Autodesk Inventor part; units mm, degrees
ref_plane "YZ Plane" through (0, 0, 0) normal (1, 0, 0) x (0, 1, 0)
ref_plane "XZ Plane" through (0, 0, 0) normal (0, 1, 0) x (-1, 0, 0)
ref_plane "XY Plane" through (0, 0, 0) normal (0, 0, 1) x (1, 0, 0)
sketch "Sketch1" plane through (0, 0, 0) normal (0, 0, 1) x (1, 0, 0)
  line L0 (-20, -7.5) -> (20, -7.5)
  line L1 (20, -7.5) -> (20, 2.5)
  line L2 (-20, 2.5) -> (-20, -7.5)
  line L3 (-17, -2.5) -> (-17, 2.5)
  line L4 (17, 2.5) -> (17, -2.5)
  line L5 (-21.1547, 2.5) -> (25.819, 2.5)
  line L6 (-17, -2.5) -> (17, -2.5)
  point P0 (0, 0)
  point P1 (0, -7.5)
  dimension "d2" = 3
  dimension "d7" = 40
  dimension "d8" = 3
  dimension "d9" = 10
  dimension "d10" = 5
  dimension "d17" = 34
  dimension "d18" = 5
extrude "Extrusion3" add sketch "Sketch1" along normal blind 200 contours L2 L5 L3 L6 L4 L1 L0
fillet "Fillet3" radius 5 1 edges at (-17, -2.5, 100)
fillet "Fillet4" radius 5 1 edges at (17, -2.5, 100)
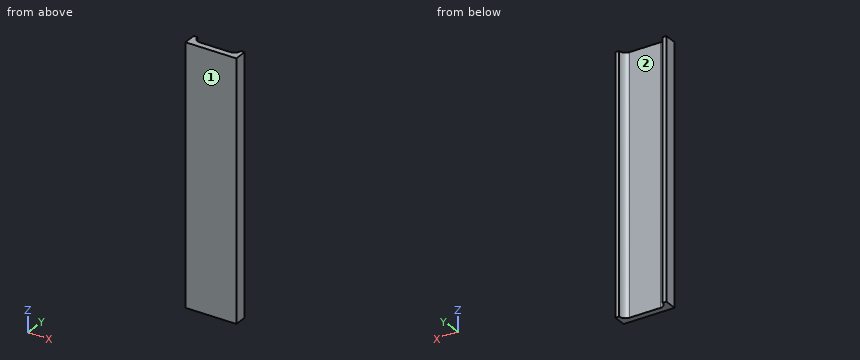
Model file for the job. Use its own axes, mm. Face numbers are marked on the shaded views. Give positions to 0.01 mm unless a question says otherwise; leave off trailing zeros. Write each loop counter-clockwise with the first axis right and the second up, starting at its lowest first coordinate (ties: lowest second). Pieces come first, ordered by that corner, then holes. Notation, with made-up numbers: (-39.75, 80.25) - (6.25, 80.25) arc R15 cw to (6.25, 99.25) - close; hole circle Ø3 at (48, 24.25). An arc over 180 degrees is marked (long way). One line per question, with ' | ' between items. Start each with the question number.
(1) Wall check: line 1 along Y through (x, z) = (3, 149); line 2 along X through (y, z) = (1.25, 126.5); line 3 along X through (y, z) = (-2, 170.5). Give the ranges that are in metal, low to high. Write a range as from..to.
(2) Pin check, flat tips, straight feed: P1, Ø19, axis at x = 4.5, z = 93, coming from the +Y side; P2, Ø1, axis at x = 16, z = 46, coming from the +Y side; P3, Ø4, axis at x = 8, z = 119.5, coming from the +Y side. Stop position of each tip, or through.
(3) Slice it at C-C on x = 1. Write the cut outline in (y, z), plus the area to 3 significant figures.
(4) Slice it at A-A on y = -0.5. Write the cut outline in (x, z), plus the area to 3 significant figures.
(5) Two-plate mould, pull along X, no slides. Class the marked faces 1 and 2: +X half, -X half, draft (parallel to the pull), parting line (faces both ways), or undercut.
(6) Slice it at D-D on x = 15. Write the cut outline in (y, z).
Results below:
1) line 1: -7.5..-2.5 | line 2: -20..-16.84, 16.84..20 | line 3: -20..-14.18, 14.18..20
2) P1: y = -2.08 | P2: y = 0.32 | P3: y = -2.5
3) outline: (-7.5, 0) - (-2.5, 0) - (-2.5, 200) - (-7.5, 200) - close | area: 1,000 mm^2
4) outline: (-20, 0) - (-16, 0) - (-16, 200) - (-20, 200) - close; (16, 0) - (20, 0) - (20, 200) - (16, 200) - close | area: 1,600 mm^2
5) face 1: draft | face 2: undercut
6) outline: (-7.5, 0) - (-1.5, 0) - (-1.5, 200) - (-7.5, 200) - close
